from build123d import *

# Parameters (mm, degrees)
EXTRUDE1_DEPTH      = 2
EXTRUDE2_DEPTH      = 299.063172834
EXTRUDE2_DEPTH_BACK = 299.063172834
SKETCH4_R           = 9.3
EXTRUDE3_DEPTH      = 0.1
CHAMFER1_SIZE       = 0.5


with BuildPart() as part:
    # Sketch1 → Revolve1 (revolve)
    with BuildSketch(Plane(origin=(0, 0, 0), x_dir=(1, 0, 0), z_dir=(0, 1, 0))):
        with BuildLine():
            Line((-11.712232269, -5.525044369), (-5.45, -18.8))
            Line((-5.45, -18.8), (-5.45, -23))
            Line((-5.45, -23), (-4, -23))
            Line((-4, -23), (-4, -292))
            Line((-4, -292), (-6.35, -292))
            Line((-6.35, -292), (-8, -293.65))
            Line((-8, -293.65), (-8, -294.9))
            ThreePointArc((-8, -294.9), (-7.238477631, -296.738477631), (-5.4, -297.5))
            Line((-5.4, -297.5), (-4.5, -297.5))
            Line((-4.5, -297.5), (-4.1, -297.1))
            Line((-4.1, -297.1), (0, -297.1))
            Line((0, -297.1), (0, -8))
            ThreePointArc((0, -8), (-8, 0), (0, 8))
            Line((0, 8), (0, 12.95))
            ThreePointArc((0, 12.95), (-10.937363132, 6.933728269), (-11.712232269, -5.525044369))
        make_face()
    revolve(axis=Axis((0, 0, 0), (0, 0, 1)))

    # Sketch2 → Extrude1 (cut)
    with BuildSketch(Plane.XY.offset(297.1)):
        Polygon((1.38672922, 0.400394061), (0.346613181, 1.401139763), (-1.040116039, 1.000745702), (-1.38672922, -0.400394061), (-0.346613181, -1.401139763), (1.040116039, -1.000745702), align=None)
    extrude(amount=-EXTRUDE1_DEPTH, mode=Mode.SUBTRACT)

    # Sketch3 → Extrude2 (cut, two sides: drawn at the far end of the back side and taken through both)
    with BuildSketch(Plane(origin=(0, 0, 0), x_dir=(0, 0, -1), z_dir=(1, 0, 0)).offset(-EXTRUDE2_DEPTH_BACK)):
        with BuildLine():
            Line((18.703975577, 4.55), (-11.6, 4.55))
            ThreePointArc((-11.6, 4.55), (-15.228015987, 4.775872106), (-18.8, 5.45))
            Line((-18.8, 5.45), (-23, 5.45))
            Line((-23, 5.45), (-23, 17.731418952))
            Line((-23, 17.731418952), (18.703975577, 17.731418952))
            Line((18.703975577, 17.731418952), (18.703975577, 4.55))
        make_face()
        with BuildLine():
            Line((18.703975577, -17.731418952), (18.703975577, -4.55))
            Line((18.703975577, -4.55), (-11.6, -4.55))
            ThreePointArc((-11.6, -4.55), (-15.228015987, -4.775872106), (-18.8, -5.45))
            Line((-18.8, -5.45), (-23, -5.45))
            Line((-23, -5.45), (-23, -17.731418952))
            Line((-23, -17.731418952), (18.703975577, -17.731418952))
        make_face()
    extrude(amount=EXTRUDE2_DEPTH + EXTRUDE2_DEPTH_BACK, mode=Mode.SUBTRACT)

    # Sketch4 → Extrude3 (cut)
    with BuildSketch(Plane(origin=(0, 4.55, 0), x_dir=(1, 0, 0), z_dir=(0, 1, 0))):
        with Locations(Location((0, 0, 0), (0, 0, 270))):
            Circle(SKETCH4_R)
    extrude3 = extrude(amount=-EXTRUDE3_DEPTH, mode=Mode.SUBTRACT)

    # Mirror1: Extrude3 across plane
    add(extrude3.mirror(Plane.ZX), mode=Mode.SUBTRACT)

    # Chamfer1
    # the kernel refuses this chamfer: 0.5, 0.360421404 mm, written as the material it takes off along each edge
    with BuildSketch(Plane(origin=(0, 4.45, 0), x_dir=(0, 0, 1), z_dir=(-1, 0, 0))) as chamfer1_piece_1:
        with BuildLine():
            Line((6.648120035 + CHAMFER1_SIZE, 0), (6.842696069, -0.305423966))
            ThreePointArc((6.842696069, -0.305423966), (6.748300889, -0.153439154), (6.648120035, 0))
            Line((6.648120035, 0), (6.648120035 + CHAMFER1_SIZE, 0))
        make_face()
    revolve(axis=Axis((0, 4.45, 0), (0, 1, 0)), mode=Mode.SUBTRACT)
    with BuildSketch(Plane(origin=(0, -4.45, 0), x_dir=(0, 0, 1), z_dir=(-1, 0, 0))) as chamfer1_piece_2:
        with BuildLine():
            Line((6.648120035 + CHAMFER1_SIZE, 0), (6.842696069, 0.305423966))
            ThreePointArc((6.842696069, 0.305423966), (6.748300889, 0.153439154), (6.648120035, 0))
            Line((6.648120035, 0), (6.648120035 + CHAMFER1_SIZE, 0))
        make_face()
    revolve(axis=Axis((0, -4.45, 0), (0, 1, 0)), mode=Mode.SUBTRACT)


solid = part.part
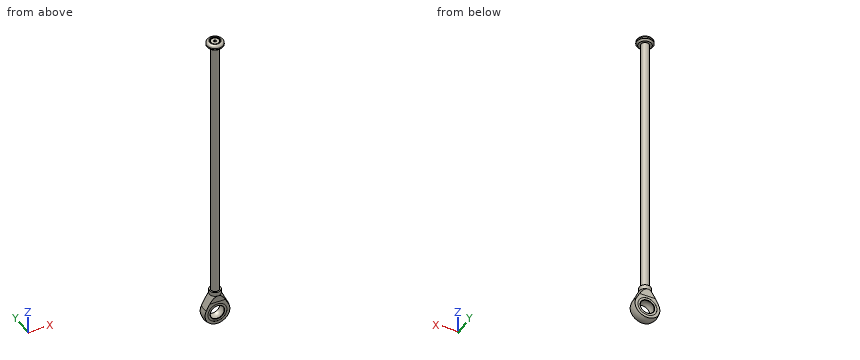
CAD build for the part. Positions are in the model's coordinates, mm. Coordinates: 2 decimals unless noted, no trailing zeros. Loops run counter-clockwise (first coordinate to the right, second up) from the corner with the lowest first, then second, coordinate; pieces in that order, holes last. Notation, with made-up numbers: (-30, 71) - (13, 71) arc R38 cw to (13, 109) - close; hole circle Ø7 at (31, 73.25). An arc over 180 degrees is marked (long way). Use one line per item in the form item = value. Start each with the question number.
1) Flat gauge pins, fed straight in: pin 1 (2 mm diameter, centred on y = -2.5, z = 135.5, fed in from -X); pin 2 (1 mm diameter, centred on x = 7, y = 1, fed in from +Z); pin 3 (1 mm diameter, centred on y = 4, z = 123, fed in from +X). Where does each tip first touch, or does it go through?
2) Band-saw the part on B-B (z = 108.5). Give the cut face in (x, y), and give its area (3 significant figures).
3) Drill centre lines: L1, parallel to X at y = 4.5, z = 0; L2, parallel to Z at x = -3.75, y = -1.75; L3, parallel to Z at x = -3, y = -4.25. Where is each one in solid material? Low to high. Write a range as from..to.
4) Band-saw the part on A-A (z = 0). Give the cut face in (x, y).
Check values:
q1.pin_1 = -3.71
q1.pin_2 = 297.22
q1.pin_3 = 1.94
q2.outline = circle Ø8 at (0, 0)
q2.area = 50.3 mm2
q3.L1 = -12.14..-9.3, 9.3..12.14
q3.L2 = -12.27..-6.85, 6.85..23, 292..297.14
q3.L3 = -11.86..-6.27, 6.27..23, 292..297.5
q4.outline = (-12.12, -4.55) - (-9.3, -4.55) - (-9.3, -4.45) - (-7.15, -4.45) - (-6.84, -4.14) arc R8 cw to (-6.84, 4.14) - (-7.15, 4.45) - (-9.3, 4.45) - (-9.3, 4.55) - (-12.12, 4.55) arc R12.95 ccw to start; (6.84, -4.14) - (7.15, -4.45) - (9.3, -4.45) - (9.3, -4.55) - (12.12, -4.55) arc R12.95 ccw to (12.12, 4.55) - (9.3, 4.55) - (9.3, 4.45) - (7.15, 4.45) - (6.84, 4.14) arc R8 cw to start
